from build123d import *

# Parameters (mm, degrees)
F1_DEPTH     = 4.5
F2_R         = 1
F4_DEPTH     = 4
F5_W         = 12.5
F5_H         = 2.9783394848
F6_DEPTH     = 3.1
F7_T1_DEPTH  = 22
F7_T3_DEPTH  = 9
F7_T6_ANGLE  = 90
F7_T10_DEPTH = 22
F7_T16_DEPTH = 22
F7_T22_DEPTH = 22
F7_T26_ANGLE = 90
F7_T30_ANGLE = 90
F7_T36_ANGLE = 90
F7_T42_ANGLE = 90
F7_T46_ANGLE = 90
F8_W         = 1
F8_H         = 5
F8_W_2       = 2
F8_W_3       = 5
F8_H_2       = 0.5
F9_DEPTH     = 2


# Not quite as in the source:
# - a fillet or chamfer that OpenCascade refuses, or shapes differently, is made with other operations: its cross-section is extruded or revolved along the edge and cut away or added


with BuildPart() as f1:
    # F0 (on Top) → F1 (new body)
    with BuildSketch(Plane.XY):
        with BuildLine():
            ThreePointArc((0, 3.8761399509), (0.2928932188, 3.1690331698), (1, 2.8761399509))
            Line((1, 2.8761399509), (26, 2.8761399509))
            ThreePointArc((26, 2.8761399509), (26.7071067812, 3.1690331698), (27, 3.8761399509))
            Line((27, 3.8761399509), (27, 13.8761399509))
            ThreePointArc((27, 13.8761399509), (26.7071067812, 14.5832467321), (26, 14.8761399509))
            Line((26, 14.8761399509), (1, 14.8761399509))
            ThreePointArc((1, 14.8761399509), (0.2928932188, 14.5832467321), (0, 13.8761399509))
            Line((0, 13.8761399509), (0, 3.8761399509))
        make_face()
        with BuildLine():
            ThreePointArc((3, 10.6761399509), (3.2928932188, 11.3832467321), (4, 11.6761399509))
            Line((4, 11.6761399509), (10.4, 11.6761399509))
            ThreePointArc((10.4, 11.6761399509), (11.1071067812, 11.3832467321), (11.4, 10.6761399509))
            Line((11.4, 10.6761399509), (11.4, 9.8761399509))
            ThreePointArc((11.4, 9.8761399509), (11.1071067812, 9.1690331698), (10.4, 8.8761399509))
            Line((10.4, 8.8761399509), (4, 8.8761399509))
            ThreePointArc((4, 8.8761399509), (3.2928932188, 9.1690331698), (3, 9.8761399509))
            Line((3, 9.8761399509), (3, 10.6761399509))
        make_face(mode=Mode.SUBTRACT)
    extrude(amount=F1_DEPTH)

    # F2
    f2_edges = [f1.edges().sort_by_distance(p)[0] for p in [
        (0.292893, 3.169033, 4.5),
        (13.5, 2.87614, 4.5),
        (26.707107, 3.169033, 4.5),
        (27, 8.87614, 4.5),
        (26.707107, 14.583247, 4.5),
        (13.5, 14.87614, 4.5),
        (0.292893, 14.583247, 4.5),
        (0, 8.87614, 4.5),
        (3.292893, 11.383247, 4.5),
        (7.2, 11.67614, 4.5),
        (11.107107, 11.383247, 4.5),
        (11.4, 10.27614, 4.5),
        (11.107107, 9.169033, 4.5),
        (7.2, 8.87614, 4.5),
        (3.292893, 9.169033, 4.5),
        (3, 10.27614, 4.5),
    ]]
    fillet(f2_edges, radius=F2_R)

    # F3 (on Top) → F4 (cut)
    with BuildSketch(Plane.XY):
        with BuildLine():
            ThreePointArc((25, 13.3761399509), (24.7071067812, 14.0832467321), (24, 14.3761399509))
            Line((24, 14.3761399509), (2, 14.3761399509))
            ThreePointArc((2, 14.3761399509), (1.2928932188, 14.0832467321), (1, 13.3761399509))
            Line((1, 13.3761399509), (1, 4.3761399509))
            ThreePointArc((1, 4.3761399509), (1.2928932188, 3.6690331698), (2, 3.3761399509))
            Line((2, 3.3761399509), (14.5, 3.3761399509))
            Line((14.5, 3.3761399509), (24, 3.3761399509))
            ThreePointArc((24, 3.3761399509), (24.7071067812, 3.6690331698), (25, 4.3761399509))
            Line((25, 4.3761399509), (25, 13.3761399509))
        make_face()
    extrude(amount=F4_DEPTH, mode=Mode.SUBTRACT)

    # F5 (on Top) → F6 (cut)
    with BuildSketch(Plane.XY):
        with Locations((18.25, 14.7778680548)):
            Rectangle(F5_W, F5_H)
    extrude(amount=F6_DEPTH, mode=Mode.SUBTRACT)

    # F7: fillet of radius 1 on 8 edges, made by hand

    # F7_s2 → F7_t1 (join)
    with BuildSketch(Plane.YZ.offset(2)):
        with BuildLine():
            ThreePointArc((3.3761399509, 3), (3.6690331698, 3.7071067812), (4.3761399509, 4))
            Line((4.3761399509, 4), (3.3761399509, 4))
            Line((3.3761399509, 4), (3.3761399509, 3))
        make_face()
    extrude(amount=F7_T1_DEPTH)

    # F7_s4 → F7_t3 (join)
    with BuildSketch(Plane.XZ.offset(-13.3761399509)):
        with BuildLine():
            ThreePointArc((25, 3), (24.7071067812, 3.7071067812), (24, 4))
            Line((24, 4), (25, 4))
            Line((25, 4), (25, 3))
        make_face()
        with BuildLine():
            ThreePointArc((1, 3), (1.2928932188, 3.7071067812), (2, 4))
            Line((2, 4), (1, 4))
            Line((1, 4), (1, 3))
        make_face()
    extrude(amount=F7_T3_DEPTH)

    # F7_s5 → F7_t6 (revolve)
    with BuildSketch(Plane.XZ.offset(-4.3761399509)):
        with BuildLine():
            ThreePointArc((1, 3), (1.2928932188, 3.7071067812), (2, 4))
            Line((2, 4), (1, 4))
            Line((1, 4), (1, 3))
        make_face()
    revolve(axis=Axis((2, 4.3761399509, 4), (0, 0, 1)), revolution_arc=F7_T6_ANGLE)


with BuildPart() as f7_tool8:
    # F7_s9 → F7_t10 (new body)
    with BuildSketch(Plane.YZ.offset(24)):
        with BuildLine():
            ThreePointArc((14.3761399509, 3), (14.0832467321, 3.7071067812), (13.3761399509, 4))
            Line((13.3761399509, 4), (14.3761399509, 4))
            Line((14.3761399509, 4), (14.3761399509, 3))
        make_face()
    extrude(amount=-F7_T10_DEPTH)

    split(bisect_by=Plane.YZ.offset(12), keep=Keep.TOP)

    split(bisect_by=Plane.XY.offset(3.1), keep=Keep.TOP)


with BuildPart() as f1_1:
    add(f1.part)

    # F7_t7: union F7_tool8
    add(f7_tool8.part)


with BuildPart() as f7_tool14:
    # F7_s15 → F7_t16 (new body)
    with BuildSketch(Plane.YZ.offset(24)):
        with BuildLine():
            ThreePointArc((14.3761399509, 3), (14.0832467321, 3.7071067812), (13.3761399509, 4))
            Line((13.3761399509, 4), (14.3761399509, 4))
            Line((14.3761399509, 4), (14.3761399509, 3))
        make_face()
    extrude(amount=-F7_T16_DEPTH)

    split(bisect_by=Plane.YZ.offset(12), keep=Keep.BOTTOM)

    split(bisect_by=Plane.XY.offset(3.1), keep=Keep.BOTTOM)


with BuildPart() as f1_2:
    add(f1_1.part)

    # F7_t13: union F7_tool14
    add(f7_tool14.part)


with BuildPart() as f7_tool20:
    # F7_s21 → F7_t22 (new body)
    with BuildSketch(Plane.YZ.offset(24)):
        with BuildLine():
            ThreePointArc((14.3761399509, 3), (14.0832467321, 3.7071067812), (13.3761399509, 4))
            Line((13.3761399509, 4), (14.3761399509, 4))
            Line((14.3761399509, 4), (14.3761399509, 3))
        make_face()
    extrude(amount=-F7_T22_DEPTH)

    split(bisect_by=Plane.YZ.offset(12), keep=Keep.BOTTOM)

    split(bisect_by=Plane.XY.offset(3.1), keep=Keep.TOP)


with BuildPart() as f1_3:
    add(f1_2.part)

    # F7_t19: union F7_tool20
    add(f7_tool20.part)

    # F7_s25 → F7_t26 (revolve)
    with BuildSketch(Plane.YZ.offset(2)):
        with BuildLine():
            ThreePointArc((14.3761399509, 3), (14.0832467321, 3.7071067812), (13.3761399509, 4))
            Line((13.3761399509, 4), (14.3761399509, 4))
            Line((14.3761399509, 4), (14.3761399509, 3))
        make_face()
    revolve(axis=Axis((2, 13.3761399509, 4), (0, 0, 1)), revolution_arc=F7_T26_ANGLE)


with BuildPart() as f7_tool28:
    # F7_s29 → F7_t30 (revolve)
    with BuildSketch(Plane.XZ.offset(-13.3761399509)):
        with BuildLine():
            ThreePointArc((25, 3), (24.7071067812, 3.7071067812), (24, 4))
            Line((24, 4), (25, 4))
            Line((25, 4), (25, 3))
        make_face()
    revolve(axis=Axis((24, 13.3761399509, 4), (0, 0, 1)), revolution_arc=F7_T30_ANGLE)

    split(bisect_by=Plane.YZ.offset(24.5), keep=Keep.TOP)

    split(bisect_by=Plane.XY.offset(3.1), keep=Keep.BOTTOM)


with BuildPart() as f1_4:
    add(f1_3.part)

    # F7_t27: union F7_tool28
    add(f7_tool28.part)


with BuildPart() as f7_tool34:
    # F7_s35 → F7_t36 (revolve)
    with BuildSketch(Plane.XZ.offset(-13.3761399509)):
        with BuildLine():
            ThreePointArc((25, 3), (24.7071067812, 3.7071067812), (24, 4))
            Line((24, 4), (25, 4))
            Line((25, 4), (25, 3))
        make_face()
    revolve(axis=Axis((24, 13.3761399509, 4), (0, 0, 1)), revolution_arc=F7_T36_ANGLE)

    split(bisect_by=Plane.YZ.offset(24.5), keep=Keep.TOP)

    split(bisect_by=Plane.XY.offset(3.1), keep=Keep.TOP)


with BuildPart() as f1_5:
    add(f1_4.part)

    # F7_t33: union F7_tool34
    add(f7_tool34.part)


with BuildPart() as f7_tool40:
    # F7_s41 → F7_t42 (revolve)
    with BuildSketch(Plane.XZ.offset(-13.3761399509)):
        with BuildLine():
            ThreePointArc((25, 3), (24.7071067812, 3.7071067812), (24, 4))
            Line((24, 4), (25, 4))
            Line((25, 4), (25, 3))
        make_face()
    revolve(axis=Axis((24, 13.3761399509, 4), (0, 0, 1)), revolution_arc=F7_T42_ANGLE)

    split(bisect_by=Plane.YZ.offset(24.5), keep=Keep.BOTTOM)

    split(bisect_by=Plane.XY.offset(3.1), keep=Keep.TOP)


with BuildPart() as f1_6:
    add(f1_5.part)

    # F7_t39: union F7_tool40
    add(f7_tool40.part)

    # F7_s45 → F7_t46 (revolve)
    with BuildSketch(Plane.YZ.offset(24)):
        with BuildLine():
            ThreePointArc((3.3761399509, 3), (3.6690331698, 3.7071067812), (4.3761399509, 4))
            Line((4.3761399509, 4), (3.3761399509, 4))
            Line((3.3761399509, 4), (3.3761399509, 3))
        make_face()
    revolve(axis=Axis((24, 4.3761399509, 4), (0, 0, 1)), revolution_arc=F7_T46_ANGLE)

    # F8 (on face) → F9 (cut)
    with BuildSketch(Plane(origin=(0, 0, 0), x_dir=(1, 0, 0), z_dir=(0, 0, -1))):
        with Locations((0.5, -8.8761399509)):
            Rectangle(F8_W, F8_H)
        with Locations((26, -8.8761399509)):
            Rectangle(F8_W_2, F8_H)
        with Locations((8.5, -3.1261399509)):
            Rectangle(F8_W_3, F8_H_2)
        with Locations((18.5, -3.1261399509)):
            Rectangle(F8_W_3, F8_H_2)
        with Locations((8.5, -14.6261399509)):
            Rectangle(F8_W_3, F8_H_2)
    extrude(amount=-F9_DEPTH, mode=Mode.SUBTRACT)


solid = f1_6.part
The model under review builds one solid part; all positions refer to its coordinate system, in mm. A direction names the side the tool comes from. Give positions to 0.01 mm unless a question says otherwise; leave off trailing zeros. Write each loop counter-clockwise with the first axis right and the second up, starting at its lowest first coordinate (ties: lowest second). Pieces come first, ordered by that corner, then holes.
1. Add section D-D, the plane y = 13. Write out the cut boundary in (x, z).
2. Draft analysis for pull direction X (two halves, no side actions). For faces 1 (the cylindrical face through (0.285, 8.806, 4.199)), 2 (the flat face through (0.5, 11.376, 1)), 3 (the cylindrical face through (7.245, 12.17, 4.362)), 4 (the cylindrical face through (13.15, 14.09, 3.7)), state which applies: +X half, -X half, draft (parallel to the pull), parting line (faces both ways), or undercut.
3. For P1, Ø0.6, axis at x = 9, y = 3, coming from the -Z side; P2, Ø0.5, axis at x = 0.5, z = 1, coming from the -Y side; P3, Ø7, axis at x = 13, y = 9.5, coming from the -Z side, all flat-tipped, find the tip position at first contact; note any pin that passes through.
4. Add section C-C, the plane x = 16.5. Write out the cut boundary in (y, z), plus the area to 3 significant figures.
5. Tool access review of faces 5 (the cylindrical face through (0.285, 3.177, 1.726)), 6 (the flat face through (25.3, 4.3, 0)), 7 (the flat face through (0.5, 8.8, 2)), 8 (the cylindrical face through (7.155, 8.382, 4.362)), 9 (the flat face through (5.96, 14.376, 2.15)): name each direction out of +Z, -Z, +X, -X, +Y, -Y from which nothing blocks a thin tool from reaching the whole face with its end or side.
6. Wall thickness on L1, parallel to Y at x = 3, z = 1.2; L2, parallel to X at y = 12.25, z = 2.85; L3, parallel to Z at x = 19, y = 5: over which ranges is each line inside the solid? List them lowest first.
7. Add section B-B, the plane z = 2.75. Write out the cut boundary in (x, y), plus the area to 3 significant figures.
8. Add section A-A, the plane x = 8. Write out the cut boundary in (y, z).
Worked answers:
1. outline: (0, 0) - (1, 0) - (1, 3) arc R1 cw to (2, 4) - (24, 4) arc R1 cw to (25, 3) - (25, 0) - (27, 0) - (27, 3.5) arc R1 ccw to (26, 4.5) - (1, 4.5) arc R1 ccw to (0, 3.5) - close
2. face 1: -X half
2. face 2: draft
2. face 3: undercut
2. face 4: undercut
3. P1: stops at z = 2
3. P2: stops at y = 2.91
3. P3: stops at z = 4
4. outline: (2.88, 2) - (3.38, 2) - (3.38, 3) arc R1 cw to (4.38, 4) - (13.38, 4) arc R1 cw to (14.37, 3.1) - (14.88, 3.1) - (14.88, 3.5) arc R1 ccw to (13.88, 4.5) - (3.88, 4.5) arc R1 ccw to (2.88, 3.5) - close
4. area: 7.45 mm2
5. face 5: +Z, -Z, -X, -Y
5. face 6: -Z, +X, -X, +Y, -Y
5. face 7: -Z, +X, -X
5. face 8: +Z
5. face 9: -Z
6. L1: y = 2.88 to 3.38, 14.38 to 14.88
6. L2: x = 0 to 1, 25 to 27
6. L3: z = 4 to 4.5
7. outline: (0, 3.88) arc R1 ccw to (1, 2.88) - (26, 2.88) arc R1 ccw to (27, 3.88) - (27, 13.88) arc R1 ccw to (26, 14.88) - (24.5, 14.88) - (24.5, 14.24) arc R1 cw to (25, 13.38) - (25, 4.38) arc R1 cw to (24, 3.38) - (2, 3.38) arc R1 cw to (1, 4.38) - (1, 13.38) arc R1 cw to (2, 14.38) - (12, 14.38) - (12, 14.88) - (1, 14.88) arc R1 ccw to (0, 13.88) - close
7. area: 53.7 mm2
8. outline: (2.88, 2) - (3.38, 2) - (3.38, 3) arc R1 cw to (4.38, 4) - (8.74, 4) arc R1 ccw to (7.88, 4.5) - (3.88, 4.5) arc R1 ccw to (2.88, 3.5) - close; (11.81, 4) - (13.38, 4) arc R1 cw to (14.38, 3) - (14.38, 2) - (14.88, 2) - (14.88, 3.5) arc R1 ccw to (13.88, 4.5) - (12.68, 4.5) arc R1 ccw to start
